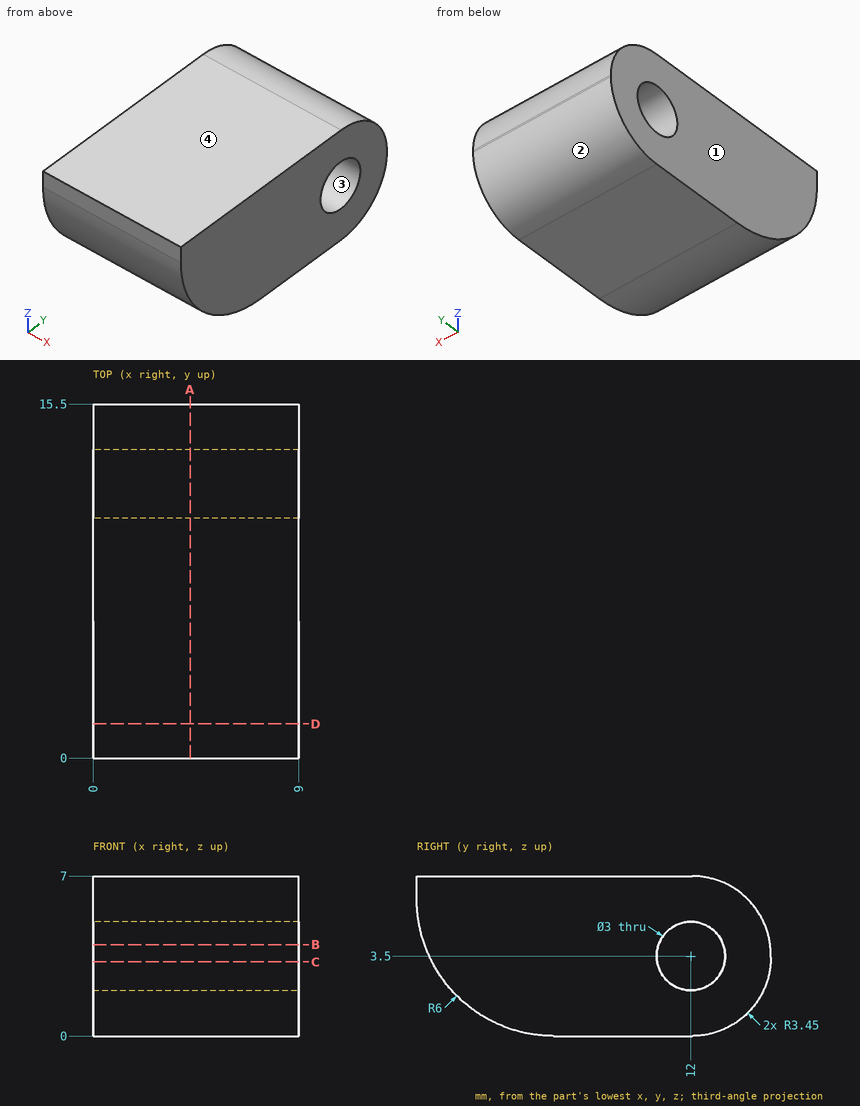
Could you check a few things on this drawing? It's one solid part, dimensions in mm from its lowest x, y, z. Coordinates: 2 decimals unless noted, no trailing zeros. Loops run counter-clockwise (first coordinate to the right, second up) from the corner with the lowest first, then second, coordinate; pieces in that order, holes last. Notation, with made-up numbers: (46, -40) - (66, -40) arc R7 cw to (66, -34) - close; hole circle Ø8 at (13.5, 50.5). An arc over 180 degrees is marked (long way). Answer as a JSON object with one key per item and string values. Group by question number.
Item 1: If I drill on L1, parallel to Z at x = 4, y = 12; L2, parallel to Y at x = 1, z = 4.5; L3, parallel to Y at x = 6.5, z = 3.5, over which ranges is the centre line in solid material (lowest first)? Write a range as from..to.
Item 2: If we section it at B-B (z = 4): List the corners of the cut face in (x, y) for me.
Item 3: If we section it at A-A (x = 4.25): List the corners of the cut face in (y, z) for me, plus the area to 3 significant figures.
Item 4: If we section it at C-C (z = 3.25): List the corners of the cut face in (x, y) for me, plus the area to 3 significant figures.
Item 5: If we section it at D-D (y = 1.5): List the corners of the cut face in (x, z) for me, plus the area to 3 significant figures.
Item 6: For pin 1 (2 mm diameter, centred on y = 2, z = 5, fed in from -X); pin 2 (1.5 mm diameter, centred on x = 2, y = 4.5, fed in from -Z); pin 3 (1.5 mm diameter, centred on x = 3.5, z = 5, fed in from -Y), each with a flat end and sliding along its axis, tell me the tip position at first contact or that it passes through.
Item 7: If we mould it in two halves opening along Z, with no side actions, what happens to the marked faces 1, 2, 3 and 4? For each: released by +Z, released by -Z, zero draft, split by the parting line, or undercut.
Returned:
{
 "1": {"L1": "z = 0..2, 5..7", "L2": "y = 0.19..10.88, 13.12..15.37", "L3": "y = 0.55..10.5, 13.5..15.5"},
 "2": {"outline": "(0, 0.34) - (9, 0.34) - (9, 10.59) - (0, 10.59) - close; (0, 13.41) - (9, 13.41) - (9, 15.47) - (0, 15.47) - close"},
 "3": {"outline": "(0, 6) arc R6 ccw to (6, 0) - (12.05, 0) arc R3.45 ccw to (15.5, 3.45) - (15.5, 3.55) arc R3.45 ccw to (12.05, 7) - (0, 7) - close; hole circle Ø3 at (12, 3.5)", "area": "88.6 mm²"},
 "4": {"outline": "(0, 0.67) - (9, 0.67) - (9, 10.52) - (0, 10.52) - close; (0, 13.48) - (9, 13.48) - (9, 15.49) - (0, 15.49) - close", "area": "107 mm²"},
 "5": {"outline": "(0, 2.03) - (9, 2.03) - (9, 7) - (0, 7) - close", "area": "44.7 mm²"},
 "6": {"pin 1": "stops at x = 0", "pin 2": "stops at z = 0.05", "pin 3": "stops at y = 0.01"},
 "7": {"face 1": "zero draft", "face 2": "released by -Z", "face 3": "undercut", "face 4": "released by +Z"}
}
